Read the model definition and answer for the solid it produces. Units are mm, in the model's axes. Face numbers are marked on the shaded views. Coordinates: 2 decimals unless noted, no trailing zeros. Order: outer loops, then holes, each group sorted by start corner. A loop starts at its lowest first (then second) coordinate and runs counter-clockwise, first axis right, second up. Notation, with made-up numbers: (-39.75, -3.75) -> (-5.75, -3.75) arc R10 cw to (-5.75, 10.25) -> close; hole circle Ø5 at (10, 30.5). An arc over 180 degrees is marked (long way). Answer as a JSON object with one key per item and string values. Group by question number.
1) Consider L1, parallel to X at y = 52.5, z = -14.5 (3 decimals); L2, parallel to Z at x = 16, y = 21 (3 decimals); L3, parallel to Y at x = 26, z = -1.5. Determine where each line is inside the solid, lowest interval first.
2) Section C-C on z = -25 is taken. Determine the outline of the cut face in (x, y) (3 decimals), and give its area (3 significant figures).
3) Section D-D on y = 23 is taken. Determine the outline of the cut face in (x, z) (3 decimals), and give its area (3 significant figures).
4) Section A-A on y = 44.45 is taken. Determine the outline of the cut face in (x, z) (3 decimals), and give its area (3 significant figures).
5) Determine the mould class of the marked faces 1, 2 and 3 for opening direction X: released by +X, released by -X, zero draft, split by the parting line, or undercut.
6) Given pin 1 (5 mm diameter, centred on y = 44.45, z = -9.525, fed in from -X); pin 2 (2.5 mm diameter, centred on x = 13.5, z = -2, fed in from +Y); pin 3 (12.5 mm diameter, centred on x = 11, y = 15, fed in from -Z) (3 decimals), each flat-ended and moving along its own axis, determine where each tip first touches the part or whether it passes through.
from build123d import *

# Parameters (mm, degrees)
SKETCH1_W                   = 31.75
SKETCH1_H                   = 31.75
SKETCH1_W_2                 = 25.4
SKETCH1_H_2                 = 25.4
BOSS_EXTRUDE1_DEPTH         = 57.15
F_1_4_0_25_DIAMETER_HOLE5_D = 6.35
SKETCH16_W                  = 25.4
SKETCH16_H                  = 57.15
CUT_EXTRUDE1_DEPTH          = 5.08
F_1_4_0_25_DIAMETER_HOLE7_D = 6.35
SKETCH20_W                  = 25.4
SKETCH20_H                  = 25.4
CUT_EXTRUDE2_DEPTH          = 5.08


with BuildPart() as part:
    # Sketch1 → Boss-Extrude1 (new body)
    with BuildSketch(Plane(origin=(0, 0, 0), x_dir=(1, 0, 0), z_dir=(0, 1, 0))):
        with Locations((15.875, 15.875)):
            Rectangle(SKETCH1_W, SKETCH1_H)
        with Locations((15.875, 15.875)):
            Rectangle(SKETCH1_W_2, SKETCH1_H_2, mode=Mode.SUBTRACT)
    extrude(amount=BOSS_EXTRUDE1_DEPTH)

    # 1/4 (0.25) Diameter Hole5 (through all)
    with Locations(Plane(origin=(31.75, 0, 0), x_dir=(0, 0, -1), z_dir=(1, 0, 0))):
        with Locations((9.525, 44.45)):
            Hole(F_1_4_0_25_DIAMETER_HOLE5_D / 2)

    # Sketch16 → Cut-Extrude1 (cut)
    with BuildSketch(Plane(origin=(0, 0, -31.75), x_dir=(-1, 0, 0), z_dir=(0, 0, -1))):
        with Locations((-15.875, 28.575)):
            Rectangle(SKETCH16_W, SKETCH16_H)
    extrude(amount=-CUT_EXTRUDE1_DEPTH, mode=Mode.SUBTRACT)

    # 1/4 (0.25) Diameter Hole7 (through all)
    with Locations(Plane.XY):
        with Locations((22.225, 6.803571429), (9.525, 15.875)):
            Hole(F_1_4_0_25_DIAMETER_HOLE7_D / 2)

    # Sketch20 → Cut-Extrude2 (cut)
    with BuildSketch(Plane.XY):
        with Locations((15.875, 44.45)):
            Rectangle(SKETCH20_W, SKETCH20_H)
    extrude(amount=-CUT_EXTRUDE2_DEPTH, mode=Mode.SUBTRACT)


solid = part.part
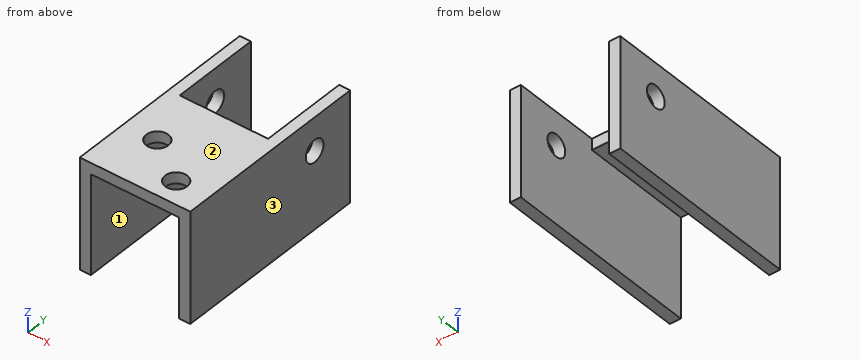
Worked answers:
{
 "1": {"L1": "x = 0 to 3.175, 28.575 to 31.75", "L2": "z = -3.175 to 0", "L3": "y = 0 to 31.75"},
 "2": {"outline": "(0, 0) -> (3.175, 0) -> (3.175, 57.15) -> (0, 57.15) -> close; (28.575, 0) -> (31.75, 0) -> (31.75, 57.15) -> (28.575, 57.15) -> close", "area": "363 mm²"},
 "3": {"outline": "(0, -31.75) -> (3.175, -31.75) -> (3.175, -3.175) -> (28.575, -3.175) -> (28.575, -31.75) -> (31.75, -31.75) -> (31.75, 0) -> (0, 0) -> close", "area": "282 mm²"},
 "4": {"outline": "(0, -31.75) -> (3.175, -31.75) -> (3.175, -12.7) -> (0, -12.7) -> close; (0, -6.35) -> (3.175, -6.35) -> (3.175, 0) -> (0, 0) -> close; (28.575, -31.75) -> (31.75, -31.75) -> (31.75, -12.7) -> (28.575, -12.7) -> close; (28.575, -6.35) -> (31.75, -6.35) -> (31.75, 0) -> (28.575, 0) -> close", "area": "161 mm²"},
 "5": {"face 1": "undercut", "face 2": "zero draft", "face 3": "released by +X"},
 "6": {"pin 1": "passes through", "pin 2": "stops at y = 31.75", "pin 3": "stops at z = -3.175"}
}
